```python
from build123d import *

# Parameters (mm, degrees)
BASE_FLANGE2_DEPTH           = 5
EDGE_FLANGE3_STRIP_W         = 26
EDGE_FLANGE3_STRIP_H         = 5
EDGE_FLANGE3_STRIP_CUT_DEPTH = 120
EDGE_FLANGE3_DEPTH           = 120
SKETCH18_R                   = 3
CUT_EXTRUDE7_DEPTH           = 10
SKETCH22_R                   = 4
CUT_EXTRUDE11_DEPTH          = 10
SKETCH25_R                   = 3.5
CUT_EXTRUDE14_DEPTH          = 10
CUT_EXTRUDE17_DEPTH          = 243.986110714
CUT_EXTRUDE17_DEPTH_BACK     = 243.986110714
SKETCH26_R                   = 3


# Sheet-metal steps are written as plain solids
with BuildPart() as part:
    # Sketch1 → Base-Flange2 (new body)
    with BuildSketch(Plane.XY):
        with BuildLine():
            Line((60, -19.74), (60, 100.5))
            ThreePointArc((60, 100.5), (58.242640687, 104.742640687), (54, 106.5))
            Line((54, 106.5), (-54, 106.5))
            ThreePointArc((-54, 106.5), (-58.242640687, 104.742640687), (-60, 100.5))
            Line((-60, 100.5), (-60, -19.74))
            Line((-60, -19.74), (60, -19.74))
        make_face()
    extrude(amount=BASE_FLANGE2_DEPTH)

    # Edge-Flange3 strip (across the edge) → Edge-Flange3 strip cut (cut)
    with BuildSketch(Plane(origin=(-60, -19.74, 5), x_dir=(0, 1, 0), z_dir=(1, 0, 0))):
        with Locations((-10, -2.5)):
            Rectangle(EDGE_FLANGE3_STRIP_W, EDGE_FLANGE3_STRIP_H)
    extrude(amount=EDGE_FLANGE3_STRIP_CUT_DEPTH, mode=Mode.SUBTRACT)

    # Edge-Flange3 section (across the edge) → Edge-Flange3 (add)
    with BuildSketch(Plane(origin=(-60, -19.74, 5), x_dir=(0, 1, 0), z_dir=(1, 0, 0))):
        with BuildLine():
            Line((-5, 3), (-5, 205))
            Line((-5, 205), (0, 205))
            Line((0, 205), (0, 3))
            ThreePointArc((0, 3), (0.878679656, 0.878679656), (3, 0))
            Line((3, 0), (3, -5))
            ThreePointArc((3, -5), (-2.656854249, -2.656854249), (-5, 3))
        make_face()
    extrude(amount=EDGE_FLANGE3_DEPTH)

    # Sketch18 → Cut-Extrude7 (cut)
    with BuildSketch(Plane.XY.offset(5)):
        with Locations((-50, 96.5)):
            Circle(SKETCH18_R)
        with Locations((50, 96.5)):
            Circle(SKETCH18_R)
    extrude(amount=-CUT_EXTRUDE7_DEPTH, mode=Mode.SUBTRACT)

    # Sketch22 → Cut-Extrude11 (cut)
    with BuildSketch(Plane(origin=(0, -19.74, 0), x_dir=(1, 0, 0), z_dir=(0, 1, 0))):
        with Locations(Location((36.205, -197, 0), (0, 0, 270))):
            Circle(SKETCH22_R)
        with Locations(Location((-36.205, -197, 0), (0, 0, 270))):
            Circle(SKETCH22_R)
        with Locations(Location((-36.205, -127, 0), (0, 0, 270))):
            Circle(SKETCH22_R)
        with Locations(Location((36.205, -127, 0), (0, 0, 270))):
            Circle(SKETCH22_R)
        with Locations(Location((36.205, -57, 0), (0, 0, 270))):
            Circle(SKETCH22_R)
        with Locations(Location((-36.205, -57, 0), (0, 0, 270))):
            Circle(SKETCH22_R)
        with Locations((60, -197)):
            Circle(SKETCH22_R)
        with Locations((60, -127)):
            Circle(SKETCH22_R)
        with Locations((-60, -197)):
            Circle(SKETCH22_R)
        with Locations((-60, -127)):
            Circle(SKETCH22_R)
        with Locations((-60, -57)):
            Circle(SKETCH22_R)
        with Locations((60, -57)):
            Circle(SKETCH22_R)
    extrude(amount=-CUT_EXTRUDE11_DEPTH, mode=Mode.SUBTRACT)

    # Sketch25 → Cut-Extrude14 (cut)
    with BuildSketch(Plane(origin=(0, 0, 0), x_dir=(-1, 0, 0), z_dir=(0, 0, -1))):
        with Locations((-47.5, -4.24)):
            Circle(SKETCH25_R)
        with Locations((47.5, -4.24)):
            Circle(SKETCH25_R)
        with BuildLine():
            ThreePointArc((16.25584062, 1.619123121), (0, 101.37), (-16.25584062, 1.619123121))
            ThreePointArc((-16.25584062, 1.619123121), (0, -9.3), (16.25584062, 1.619123121))
        make_face()
    extrude(amount=-CUT_EXTRUDE14_DEPTH, mode=Mode.SUBTRACT)

    # Sketch26 → Cut-Extrude17 (cut, two sides: drawn at the far end of the back side and taken through both)
    with BuildSketch(Plane(origin=(0, 0, 0), x_dir=(-1, 0, 0), z_dir=(0, 0, -1)).offset(-CUT_EXTRUDE17_DEPTH_BACK)):
        with BuildLine():
            Line((-60, 50.17), (-51.2, 50.17))
            ThreePointArc((-51.2, 50.17), (0, 101.37), (51.2, 50.17))
            Line((51.2, 50.17), (60, 50.17))
            Line((60, 50.17), (60, 100.5))
            ThreePointArc((60, 100.5), (58.242640687, 104.742640687), (54, 106.5))
            Line((54, 106.5), (-54, 106.5))
            ThreePointArc((-54, 106.5), (-58.242640687, 104.742640687), (-60, 100.5))
            Line((-60, 100.5), (-60, 50.17))
        make_face()
        with Locations((-50, 96.5)):
            Circle(SKETCH26_R, mode=Mode.SUBTRACT)
        with Locations((50, 96.5)):
            Circle(SKETCH26_R, mode=Mode.SUBTRACT)
    extrude(amount=CUT_EXTRUDE17_DEPTH + CUT_EXTRUDE17_DEPTH_BACK, mode=Mode.SUBTRACT)


solid = part.part
```
Geometry check sheet. Reference: the model listing, model coordinates, mm. A direction names the side the tool comes from. Round coordinates to 2 decimals unless told otherwise and drop trailing zeros. Loops run counter-clockwise (first coordinate to the right, second up) from the corner with the lowest first, then second, coordinate; pieces in that order, holes last. Notation, with made-up numbers: M -15.75,20 L 23.25,20 A25 cw 23.25,35 Z; hole C -24.5,88.25 d3. An arc over 180 degrees is marked long. Return JSON: item names as keys, results as strings. Group by question number.
(1) Section check B-B, the plane x = -47.5. Enter the section's corners in (y, z), and give its area (3 significant figures).
(2) Scan lines: line 1 along Z through (x, y) = (55.5, 34.5); line 2 along Y through (x, z) = (-50, 48); line 3 along X through (y, z) = (-4, 2). Record each from-to range of solid material in increasing order. Write a range as [from, to].
(3) Section check A-A, the plane z = 57. Enter the section's corners in (x, y) (3 decimals), and give its area (3 significant figures).
(4) Go/stop test with flat-tipped pins: pin 1 (6.5 mm diameter, centred on x = 36.205, z = 57, fed in from -Y); pin 2 (5 mm diameter, centred on x = 42.5, y = -16, fed in from +Z). Record where each tip stops, or that it passes through.
(5) Mould release check, pull along Z, two halves, no side actions. Record for faces 4 (the face through (-60, -22, 162)), 5 (the face through (-0.84, -22.334, 2.281)), 6 (the face through (37.406, -22.205, 200.815)): pulls with the +Z half, pulls with the -Z half, needs draft (parallel to the pull), parting line crosses it, or undercut.
(6) Section check D-D, the plane y = -4.24. Enter the section's corners in (x, z), and give its area (3 significant figures).
(7) Section check C-C, the plane y = 39.5. Enter the section's corners in (x, z).
(8) Set-up check for faces 1 (the face through (60, -1, 3)), 2 (the face through (-1, -19.74, 110)), 3 (the face through (41.8, 20.6, 2.5)): record each of +Z, -Z, +X, -X, +Y, -Y from which the full face is reachable in a straight line by a thin tool's end or side.
Data:
{
 "1": {"outline": "M -24.74,8 A8 ccw -16.74,0 L -7.74,0 L -7.74,5 L -16.74,5 A3 cw -19.74,8 L -19.74,210 L -24.74,210 Z; M -0.74,0 L 31.06,0 L 31.06,5 L -0.74,5 Z", "area": "1,260 mm²"},
 "2": {"line 1": "[0, 5]", "line 2": "[-24.74, -19.74]", "line 3": "[-60, -50.99], [-44.01, -12.57], [12.57, 44.01], [50.99, 60]"},
 "3": {"outline": "M -56,-24.74 L -40.205,-24.74 L -40.205,-19.74 L -56,-19.74 Z; M -32.205,-24.74 L 32.205,-24.74 L 32.205,-19.74 L -32.205,-19.74 Z; M 40.205,-24.74 L 56,-24.74 L 56,-19.74 L 40.205,-19.74 Z", "area": "480 mm²"},
 "4": {"pin 1": "through", "pin 2": "z = 5.57"},
 "5": {"face 4": "needs draft", "face 5": "pulls with the -Z half", "face 6": "undercut"},
 "6": {"outline": "M -60,0 L -51,0 L -51,5 L -60,5 Z; M -44,0 L -12.33,0 L -12.33,5 L -44,5 Z; M 12.33,0 L 44,0 L 44,5 L 12.33,5 Z; M 51,0 L 60,0 L 60,5 L 51,5 Z", "area": "407 mm²"},
 "7": {"outline": "M -60,0 L -50.08,0 L -50.08,5 L -60,5 Z; M 50.08,0 L 60,0 L 60,5 L 50.08,5 Z"},
 "8": {"face 1": "+Z, -Z, +X, +Y, -Y", "face 2": "+Z, +X, -X, +Y", "face 3": "+Z, -Z, +Y"}
}
